Can you work these out from the model? Positions are in its coordinate system, mm. Give positions to 0.01 mm unless a question says otherwise; leave off trailing zeros. Order: outer loops, then holes, each group sorted by start corner. A loop starts at its lowest first (then second) coordinate and runs counter-clockwise, first axis right, second up.
Item 1: I'm going to push flat-ended pins straight in: pin 1 Ø4 at (y, z) = (-5.5, -37.5) entering from +X; pin 2 Ø4 at (y, z) = (-6, -27) entering from +X. Where does each tip first touch, or does it pass through?
Item 2: I want a section at B-B, the plane y = -10.75. Write out the boundary of the cut face in (x, z).
Item 3: If I drill on line 1 along Y through (x, z) = (115.5, -32.5); line 2 along X through (y, z) = (-6.5, -11.5); line 3 along Y through (x, z) = (11.5, -19), over which ranges is the centre line in solid material (lowest first)?
Item 4: I want a section at A-A, the plane z = -6. Write out the boundary of the cut face in (x, y).
```python
from build123d import *

# Parameters (mm, degrees)
F0_W     = 124.714
F0_H     = 76.2
F1_DEPTH = 11.938
F3_DEPTH = 76.201
F5_DEPTH = 76.201


with BuildPart() as f1:
    # F0 (on Front) → F1 (new body)
    with BuildSketch(Plane.XZ):
        with Locations((62.357, -38.1)):
            Rectangle(F0_W, F0_H)
    extrude(amount=F1_DEPTH)

    # F2 (on face) → F3 (cut, through all)
    with BuildSketch(Plane(origin=(0, 0, -76.2), x_dir=(1, 0, 0), z_dir=(0, 0, -1))):
        Polygon((11.938, 0), (0, 11.938), (0, 0), align=None)
    extrude(amount=-F3_DEPTH, mode=Mode.SUBTRACT)

    # F4 (on face) → F5 (cut, through all)
    with BuildSketch(Plane(origin=(0, 0, -76.2), x_dir=(1, 0, 0), z_dir=(0, 0, -1))):
        Polygon((124.714, 0), (124.714, 11.938), (112.776, 0), align=None)
    extrude(amount=-F5_DEPTH, mode=Mode.SUBTRACT)


solid = f1.part
```
Results list:
1. pin 1: stops at x = 120.28
1. pin 2: stops at x = 120.78
2. outline: (1.19, -76.2) - (123.53, -76.2) - (123.53, 0) - (1.19, 0) - close
3. line 1: y = -11.94 to -2.72
3. line 2: x = 5.44 to 119.28
3. line 3: y = -11.94 to -0.44
4. outline: (0, -11.94) - (124.71, -11.94) - (112.78, 0) - (11.94, 0) - close
